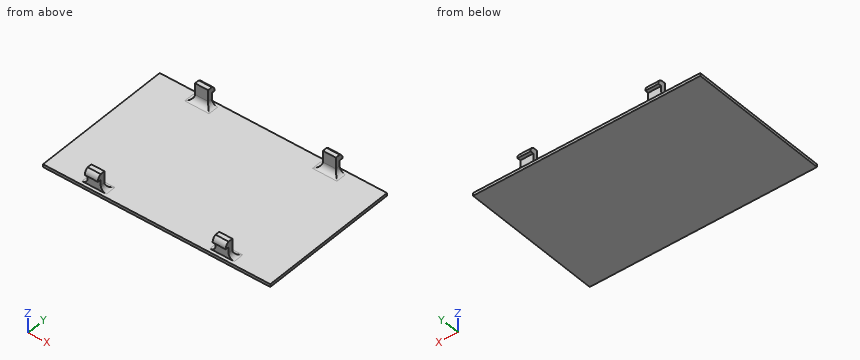
Autodesk Inventor part; units mm, degrees
ref_plane "Work Plane1" through (-0.47, 22.2, 1) normal (-1, 0, 0) x (0, 0, 1)
ref_plane "YZ Plane" through (0, 0, 0) normal (1, 0, 0) x (0, 1, 0)
ref_plane "XZ Plane" through (0, 0, 0) normal (0, 1, 0) x (-1, 0, 0)
sketch "Sketch1" plane through (0, 0, 0) normal (0, 0, 1) x (1, 0, 0)
  line L0 (0, 10.3664) -> (0, -9.7905)
  line L1 (-11.2303, 0) -> (9.7082, 0)
  line L2 (-40, 25) -> (40, 25)
  line L3 (40, 25) -> (40, -25)
  line L4 (40, -25) -> (-40, -25)
  line L5 (-40, -25) -> (-40, 25)
  point P0 (0, 0)
  dimension "d0" = 80
  dimension "d1" = 50
extrude "Extrusion1" add sketch "Sketch1" along normal blind 1
sketch "Sketch2" plane through (0, 0, 1) normal (0, 0, 1) x (1, 0, 0)
  line L0 (-25.47, 29.9826) -> (-25.47, 14.8936)
  line L1 (-40, 25) -> (-40, -25)
  line L2 (-20.47, 29.2374) -> (-20.47, 19.4575)
  line L3 (19.53, 30.5414) -> (19.53, 15.3593)
  line L4 (40, -25) -> (40, 25)
  line L5 (24.53, 28.7717) -> (24.53, 17.8741)
  line L6 (-43.5467, 24) -> (46.149, 24)
  line L7 (40, 25) -> (-40, 25)
  line L8 (-25.47, 24) -> (-20.47, 24)
  line L9 (-20.47, 24) -> (-20.47, 22)
  line L10 (-20.47, 22) -> (-25.47, 22)
  line L11 (-25.47, 22) -> (-25.47, 24)
  line L12 (-25.27, 22.2) -> (-20.67, 22.2)
  line L13 (-20.67, 22.2) -> (-20.67, 23.8)
  line L14 (-20.67, 23.8) -> (-25.27, 23.8)
  line L15 (-25.27, 23.8) -> (-25.27, 22.2)
  line L16 (19.53, 24) -> (24.53, 24)
  line L17 (24.53, 24) -> (24.53, 22)
  line L18 (24.53, 22) -> (19.53, 22)
  line L19 (19.53, 22) -> (19.53, 24)
  line L20 (19.73, 22.2) -> (24.33, 22.2)
  line L21 (24.33, 22.2) -> (24.33, 23.8)
  line L22 (24.33, 23.8) -> (19.73, 23.8)
  line L23 (19.73, 23.8) -> (19.73, 22.2)
  point P0 (0, 0)
  dimension "d4" = 14.53
  dimension "d5" = 19.53
  dimension "d6" = 20.47
  dimension "d7" = 15.47
  dimension "d8" = 1
  dimension "d9" = 4
  dimension "d10" = 0.2
  dimension "d11" = 4
  dimension "d12" = 0.2
extrude "Extrusion2" add sketch "Sketch2" along normal blind 6 contours L15 L14 L13 L12 | L23 L22 L21 L20
sketch "Sketch4" plane through (-25.27, 22.2, 1) normal (-1, 0, 0) x (0, 0, 1)
  line L0 (0, 1.6) -> (6, 1.6)
  arc A0 (6, 1.6) -> (4, 2.8) centre (4.164, 0.8067) ccw
  line L1 (6, 1.6) -> (6, 0)
  line L2 (4, 2.8) -> (4, 1.6)
  line L3 (4, 1.6) -> (6, 1.6)
  point P0 (-1, -22.2)
  dimension "d15" = 1.2
  dimension "d16" = 2
  dimension "d17" = 2
extrude "Extrusion3" add sketch "Sketch4" against normal up to surface (4.6 mm away)
ref_plane "Work Plane1" through (-0.47, 22.2, 1) normal (-1, 0, 0) x (0, 0, 1)
mirror "Mirror2" about plane through (0, 0, 0) normal (0, 1, 0) of "Extrusion3", "Extrusion2"
mirror "Mirror1" about plane through (-0.47, 22.2, 1) normal (-1, 0, 0) of "Extrusion3", "Extrusion2", "Mirror2"
fillet "Fillet1" radius 2 12 edges at (-20.67, -23, 1) (-22.97, -22.2, 1) (-25.27, -23, 1) (24.33, -23, 1) (22.03, -22.2, 1) (19.73, -23, 1) (19.73, 23, 1) (22.03, 22.2, 1) (24.33, 23, 1) (-20.67, 23, 1) (-22.97, 22.2, 1) (-25.27, 23, 1)
properties part number "cover"
Geometry check sheet. Reference: the model listing, model coordinates, mm. Round coordinates to 2 decimals unless told otherwise and drop trailing zeros. Loops run counter-clockwise (first coordinate to the right, second up) from the corner with the lowest first, then second, coordinate; pieces in that order, holes last. Notation, with made-up numbers: (54.25, -17.75) -> (103.25, -17.75) arc R32 cw to (103.25, 13.25) -> close; hole circle Ø5 at (33.5, -19). An arc over 180 degrees is marked (long way). Use a Markdown table: item, result.
(1) Sectioned sample at D-D (y = -8). Enter the section's corners in (x, z).
Calculated:
| item | result |
|---|---|
| outline | (-40, 0) -> (40, 0) -> (40, 1) -> (-40, 1) -> close |
(2) Scan lines: probe 1 along Z at (x, y) = (-31, 19); probe 2 along Y at (x, z) = (20.5, 0.75); probe 3 along Y at (x, z) = (-25, 5.75). Record each from-to range of solid material in increasing order.
Calculated:
| item | result |
|---|---|
| probe 1 | 0 to 1 |
| probe 2 | -25 to 25 |
| probe 3 | -24.92 to -22.2, 22.2 to 24.92 |
(3) Sectioned sample at B-B (y = -21). Enter the section's corners in (x, z), then the cut area to 3 significant figures.
Calculated:
| item | result |
|---|---|
| outline | (-40, 0) -> (40, 0) -> (40, 1) -> (26.33, 1) arc R2 cw to (25.53, 1.17) -> (18.53, 1.17) arc R2 cw to (17.73, 1) -> (-18.67, 1) arc R2 cw to (-19.47, 1.17) -> (-26.47, 1.17) arc R2 cw to (-27.27, 1) -> (-40, 1) -> close |
| area | 82.5 mm² |
(4) Sectioned sample at C-C (x = 13.5). Enter the section's corners in (y, z).
Calculated:
| item | result |
|---|---|
| outline | (-25, 0) -> (25, 0) -> (25, 1) -> (-25, 1) -> close |
(5) Go/stop test with flat-tipped pins: P1, Ø3, axis at x = 8, z = 2, coming from the +Y side; P2, Ø0.8, axis at y = 24, z = 5, coming from the +X side; P3, Ø1, axis at y = -6, z = 2.5, coming from the +X side; P4, Ø0.8, axis at y = -24, z = 4.5, coming from the -X side. Record where each tip stops, or that it passes through.
Calculated:
| item | result |
|---|---|
| P1 | y = 25 |
| P2 | x = 24.33 |
| P3 | through |
| P4 | x = -25.27 |
(6) Sectioned sample at A-A (z = 4). Enter the section's corners in (x, y), then the cut area to 3 significant figures.
Calculated:
| item | result |
|---|---|
| outline | (-25.27, -23.8) -> (-20.67, -23.8) -> (-20.67, -22.2) -> (-25.27, -22.2) -> close; (-25.27, 22.2) -> (-20.67, 22.2) -> (-20.67, 23.8) -> (-25.27, 23.8) -> close; (19.73, -23.8) -> (24.33, -23.8) -> (24.33, -22.2) -> (19.73, -22.2) -> close; (19.73, 22.2) -> (24.33, 22.2) -> (24.33, 23.8) -> (19.73, 23.8) -> close |
| area | 29.4 mm² |
